Build history of the part. All positions in model axes, mm. Face numbers are marked on the shaded views. Round coordinates to 2 decimals unless told otherwise and drop trailing zeros. Write each loop counter-clockwise with the first axis right and the second up, starting at its lowest first coordinate (ties: lowest second). Pieces come first, ordered by that corner, then holes. Notation, with made-up numbers: M 45,-28.5 L 80,-28.5 A11 cw 80,-13.5 Z; hole C -15,18 d11. An arc over 180 degrees is marked long. Use a Markdown table: item, result.
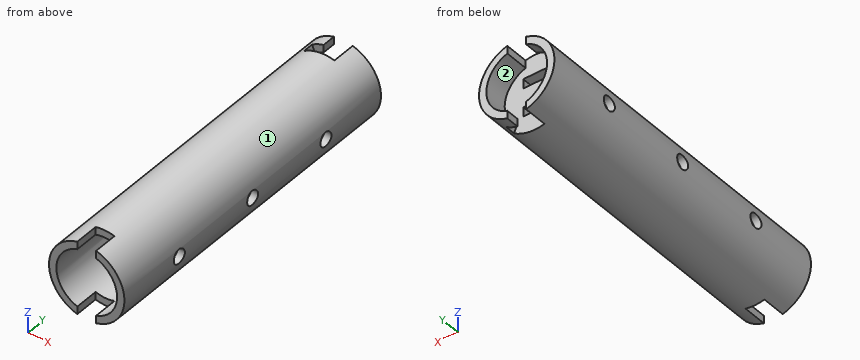
from build123d import *

# Parameters (mm, degrees)
SKETCH2_R                      = 10.16
SKETCH2_R_2                    = 8.1788
BOSS_EXTRUDE2_DEPTH            = 44.45
CUT_EXTRUDE1_DEPTH             = 6.35
CUT_EXTRUDE3_REACH             = 48.715
SKETCH5_R                      = 1.905
CUT_EXTRUDE3_DIRECTION_2_DEPTH = 13.97
CUT_EXTRUDE4_START             = -3.556
CUT_EXTRUDE4_DEPTH             = 2.794
BOSS_EXTRUDE3_START            = -2.54
SKETCH7_R                      = 8.1788
SKETCH7_W                      = 6.35
SKETCH7_H                      = 2.54
BOSS_EXTRUDE3_DEPTH            = 2.54


with BuildPart() as part:
    # Sketch2 → Boss-Extrude2 (new, symmetric)
    with BuildSketch(Plane(origin=(0, 0, 0), x_dir=(1, 0, 0), z_dir=(0, 1, 0))):
        with Locations(Location((0, 0, 0), (0, 0, 270))):
            Circle(SKETCH2_R)
        with Locations(Location((0, 0, 0), (0, 0, 270))):
            Circle(SKETCH2_R_2, mode=Mode.SUBTRACT)
    extrude(amount=BOSS_EXTRUDE2_DEPTH, both=True)

    # Sketch4 → Cut-Extrude1 (cut)
    with BuildSketch(Plane(origin=(0, 44.45, 0), x_dir=(1, 0, 0), z_dir=(0, 1, 0))):
        with BuildLine():
            Line((-2.54, 9.837377699), (-2.54, -9.837377699))
            ThreePointArc((-2.54, -9.837377699), (0, -10.16), (2.54, -9.837377699))
            Line((2.54, -9.837377699), (2.54, 9.837377699))
            ThreePointArc((2.54, 9.837377699), (0, 10.16), (-2.54, 9.837377699))
        make_face()
    cut_extrude1 = extrude(amount=-CUT_EXTRUDE1_DEPTH, mode=Mode.SUBTRACT)

    # Mirror1: Cut-Extrude1 across plane
    add(cut_extrude1.mirror(Plane.ZX), mode=Mode.SUBTRACT)

    # Sketch5 → Cut-Extrude3 (cut, up to next)
    with BuildSketch(Plane(origin=(0, 0, 0), x_dir=(0, 0, -1), z_dir=(1, 0, 0)), mode=Mode.PRIVATE) as cut_extrude3_sk1:
        with Locations(Location((0, 0, 0), (0, 0, 180))):
            Circle(SKETCH5_R)
    cut_extrude3_tool1 = extrude(cut_extrude3_sk1.sketch, amount=-CUT_EXTRUDE3_REACH, mode=Mode.PRIVATE) & part.part
    # Sketch5 → Cut-Extrude3 (cut, up to next)
    with BuildSketch(Plane(origin=(0, 0, 0), x_dir=(0, 0, -1), z_dir=(1, 0, 0)), mode=Mode.PRIVATE) as cut_extrude3_sk2:
        with Locations(Location((0, 25.4, 0), (0, 0, 180))):
            Circle(SKETCH5_R)
    cut_extrude3_tool2 = extrude(cut_extrude3_sk2.sketch, amount=-CUT_EXTRUDE3_REACH, mode=Mode.PRIVATE) & part.part
    # Sketch5 → Cut-Extrude3 (cut, up to next)
    with BuildSketch(Plane(origin=(0, 0, 0), x_dir=(0, 0, -1), z_dir=(1, 0, 0)), mode=Mode.PRIVATE) as cut_extrude3_sk3:
        with Locations((0, -25.4)):
            Circle(SKETCH5_R)
    cut_extrude3_tool3 = extrude(cut_extrude3_sk3.sketch, amount=-CUT_EXTRUDE3_REACH, mode=Mode.PRIVATE) & part.part
    add(cut_extrude3_tool1.solids().sort_by_distance((0, 0, 0))[0], mode=Mode.SUBTRACT)
    add(cut_extrude3_tool2.solids().sort_by_distance((0, 25.4, 0))[0], mode=Mode.SUBTRACT)
    add(cut_extrude3_tool3.solids().sort_by_distance((0, -25.4, 0))[0], mode=Mode.SUBTRACT)

    # Sketch5 → Cut-Extrude3 direction 2 (cut)
    with BuildSketch(Plane(origin=(0, 0, 0), x_dir=(0, 0, -1), z_dir=(1, 0, 0))):
        with Locations(Location((0, 0, 0), (0, 0, 180))):
            Circle(SKETCH5_R)
        with Locations(Location((0, 25.4, 0), (0, 0, 180))):
            Circle(SKETCH5_R)
        with Locations((0, -25.4)):
            Circle(SKETCH5_R)
    extrude(amount=CUT_EXTRUDE3_DIRECTION_2_DEPTH, mode=Mode.SUBTRACT)

    # Sketch6 → Cut-Extrude4 (cut)
    with BuildSketch(Plane(origin=(0, 44.45, 0), x_dir=(1, 0, 0), z_dir=(0, 1, 0)).offset(CUT_EXTRUDE4_START)):
        with BuildLine():
            Line((-4.918424262, -6.534666955), (-5.62055167, -8.463746152))
            ThreePointArc((-5.62055167, -8.463746152), (-4.137676497, -9.279290555), (-2.54, -9.837377699))
            Line((-2.54, -9.837377699), (-2.54, -7.774391902))
            ThreePointArc((-2.54, -7.774391902), (-3.78037731, -7.252690317), (-4.918424262, -6.534666955))
        make_face()
        with BuildLine():
            Line((2.54, 7.774391902), (2.54, 9.837377699))
            ThreePointArc((2.54, 9.837377699), (4.137676497, 9.279290555), (5.62055167, 8.463746152))
            Line((5.62055167, 8.463746152), (4.918424262, 6.534666955))
            ThreePointArc((4.918424262, 6.534666955), (3.78037731, 7.252690317), (2.54, 7.774391902))
        make_face()
    extrude(amount=-CUT_EXTRUDE4_DEPTH, mode=Mode.SUBTRACT)

    # Sketch7 → Boss-Extrude3 (add)
    with BuildSketch(Plane(origin=(0, 38.1, 0), x_dir=(1, 0, 0), z_dir=(0, 1, 0)).offset(BOSS_EXTRUDE3_START)):
        with Locations(Location((0, 0, 0), (0, 0, 71.907077979))):
            Circle(SKETCH7_R)
        with Locations((0, 3.81)):
            Rectangle(SKETCH7_W, SKETCH7_H, mode=Mode.SUBTRACT)
        with Locations((0, -3.81)):
            Rectangle(SKETCH7_W, SKETCH7_H, mode=Mode.SUBTRACT)
    extrude(amount=BOSS_EXTRUDE3_DEPTH)


solid = part.part
Q1. Drill centre lines: L1, parallel to Y at x = -8.65, z = 0 (3 decimals); L2, parallel to X at y = -19, z = -0.5; L3, parallel to Y at x = 0.25, z = 6.25. Where is each one in solid material? Low to high.
Response values:
| item | result |
|---|---|
| L1 | y = -44.45 to -27.305, -23.495 to -1.905, 1.905 to 23.495, 27.305 to 44.45 |
| L2 | x = -10.15 to -8.16, 8.16 to 10.15 |
| L3 | y = 35.56 to 38.1 |
Q2. Drop flat-ended pins along their axis: P1, Ø12, axis at x = 7, y = 31, coming from the +Z side; P2, Ø1, axis at y = 42.5, z = -9, coming from the +X side; P3, Ø2.5, axis at y = -39.5, z = 9, coming from the -X side. Give the stop position or say it passes through.
Response values:
| item | result |
|---|---|
| P1 | stops at z = 10.11 |
| P2 | stops at x = 5.57 |
| P3 | stops at x = -6.57 |
Q3. Cut at D-D on y = 4. Give the cut face in (x, z).
Response values:
| item | result |
|---|---|
| outline | C 0,0 d20.32; hole C 0,0 d16.36 |
Q4. Cut at A-A on z = -3.5. Give the cut face in (x, y) (3 decimals).
Response values:
| item | result |
|---|---|
| outline | M -9.538,-44.45 L -7.392,-44.45 L -7.392,35.56 L -3.175,35.56 L -3.175,38.1 L -7.392,38.1 L -7.392,44.45 L -9.538,44.45 Z; M 3.175,35.56 L 7.392,35.56 L 7.392,-44.45 L 9.538,-44.45 L 9.538,44.45 L 7.392,44.45 L 7.392,38.1 L 3.175,38.1 Z |
Q5. Cut at B-B on y = 25.4. Give the cut face in (x, z) (3 decimals), and give its area (3 significant figures).
Response values:
| item | result |
|---|---|
| outline | M -9.98,-1.905 A10.16 ccw 9.98,-1.905 L 7.954,-1.905 A8.179 cw -7.954,-1.905 Z; M -9.98,1.905 L -7.954,1.905 A8.179 cw 7.954,1.905 L 9.98,1.905 A10.16 ccw Z |
| area | 98.9 mm2 |
Q6. Two-plate mould, pull along X, no slides. Class the marked faces 1 and 2: +X half, -X half, draft (parallel to the pull), parting line (faces both ways), or undercut.
Response values:
| item | result |
|---|---|
| face 1 | parting line |
| face 2 | undercut |
Q7. Cut at C-C on z = 0. Count the separate pieces of the cut face and the enclosed holes in it, and give its area (3 significant figures).
Response values:
| item | result |
|---|---|
| separate pieces | 7 |
| enclosed holes | 0 |
| area | 349 mm2 |
